```python
from build123d import *

# Parameters (mm, degrees)
BASPROSKE_W             = 10
BASPROSKE_H             = 11
TOOTHCUT_DEPTH          = 19.493242009
TEETHCUTS_COUNT         = 20
TEETHCUTS_ANGLE         = 342
BORSKE_R                = 0.4
BORE_DEPTH              = 50.0000508
CROQUIS1_R              = 2
SALIENTE_EXTRUIR1_DEPTH = 10
CROQUIS2_R              = 2
CORTAR_EXTRUIR1_DEPTH   = 10
CORTAR_EXTRUIR2_DEPTH   = 10


with BuildPart() as part:
    # BasProSke → Base-Revolve (revolve)
    with BuildSketch(Plane(origin=(0, 0, 0), x_dir=(1, 0, 0), z_dir=(0, 1, 0)), mode=Mode.PRIVATE) as base_revolve_sk:
        with Locations((5, 5.5)):
            Rectangle(BASPROSKE_W, BASPROSKE_H)
    revolve(base_revolve_sk.sketch.rotate(Axis((-10, 0, 0), (1, 0, 0)), 180), axis=Axis((-10, 0, 0), (1, 0, 0)))

    # TooCutSke → ToothCut (cut, through all)
    with BuildSketch(Plane(origin=(0, 0, 0), x_dir=(0, 0, -1), z_dir=(1, 0, 0))):
        with BuildLine():
            ThreePointArc((0.499924007, 8.734705318), (0, 8.749), (-0.499924007, 8.734705318))
            ThreePointArc((-0.499924007, 8.734705318), (-0.824302243, 9.905497836), (-1.485192705, 10.924909509))
            ThreePointArc((-1.485192705, 10.924909509), (0, 11.0254), (1.485192705, 10.924909509))
            ThreePointArc((1.485192705, 10.924909509), (0.824302243, 9.905497836), (0.499924007, 8.734705318))
        make_face()
    toothcut = extrude(amount=TOOTHCUT_DEPTH, mode=Mode.SUBTRACT)

    # TeethCuts: ToothCut ×20 about axis
    teethcuts_axis = Axis((-10, 0, 0), (1, 0, 0))
    for i in range(1, TEETHCUTS_COUNT):
        add(toothcut.rotate(teethcuts_axis, i * TEETHCUTS_ANGLE / (TEETHCUTS_COUNT - 1)), mode=Mode.SUBTRACT)

    # BorSke → Bore (cut, symmetric)
    with BuildSketch(Plane(origin=(0, 0, 0), x_dir=(0, 0, -1), z_dir=(1, 0, 0))):
        with Locations(Location((0, 0, 0), (0, 0, 180))):
            Circle(BORSKE_R)
    extrude(amount=BORE_DEPTH, both=True, mode=Mode.SUBTRACT)

    # Croquis1 → Saliente-Extruir1 (add)
    with BuildSketch(Plane(origin=(10, 0, 0), x_dir=(0, 0, -1), z_dir=(1, 0, 0))):
        with BuildLine():
            Line((40, 5), (0, 5))
            ThreePointArc((0, 5), (-5, 0), (0, -5))
            Line((0, -5), (40, -5))
            ThreePointArc((40, -5), (45, 0), (40, 5))
        make_face()
        Circle(CROQUIS1_R, mode=Mode.SUBTRACT)
        with Locations((40, 0)):
            Circle(CROQUIS1_R, mode=Mode.SUBTRACT)
    extrude(amount=-SALIENTE_EXTRUIR1_DEPTH)

    # Croquis2 → Cortar-Extruir1 (cut)
    with BuildSketch(Plane(origin=(10, 0, 0), x_dir=(0, 0, -1), z_dir=(1, 0, 0))):
        Circle(CROQUIS2_R)
    extrude(amount=-CORTAR_EXTRUIR1_DEPTH, mode=Mode.SUBTRACT)

    # Croquis3 → Cortar-Extruir2 (cut)
    with BuildSketch(Plane(origin=(10, 0, 0), x_dir=(0, 0, -1), z_dir=(1, 0, 0))):
        with BuildLine():
            Line((6.772677084, 5.538577987), (8.515195785, 6.963579593))
            ThreePointArc((8.515195785, 6.963579593), (9.209061868, 6.016076754), (9.797958971, 5))
            Line((9.797958971, 5), (7.179484731, 5))
            ThreePointArc((7.179484731, 5), (6.981276487, 5.273213405), (6.772677084, 5.538577987))
        make_face()
        with BuildLine():
            Line((6.772677084, -5.538577987), (8.515195785, -6.963579593))
            ThreePointArc((8.515195785, -6.963579593), (9.209061868, -6.016076754), (9.797958971, -5))
            Line((9.797958971, -5), (7.179484731, -5))
            ThreePointArc((7.179484731, -5), (6.981276487, -5.273213405), (6.772677084, -5.538577987))
        make_face()
    extrude(amount=-CORTAR_EXTRUIR2_DEPTH, mode=Mode.SUBTRACT)


solid = part.part
```
Design review of the part built by this model. Coordinates are the model's own, in mm. A direction names the side the tool comes from. Round coordinates to 2 decimals unless told otherwise and drop trailing zeros. Write each loop counter-clockwise with the first axis right and the second up, starting at its lowest first coordinate (ties: lowest second). Pieces come first, ordered by that corner, then holes. Notation, with made-up numbers: (-17, 46.5) -> (4, 46.5) arc R18 cw to (4, 79.5) -> close; hole circle Ø9 at (35, -2). An arc over 180 degrees is marked (long way). Answer in a Markdown table with one row per item.
Q1. Clearance check with flat-ended pins moving along their axes: pin 1 Ø3 at (x, z) = (4, -18.5) entering from -Y; pin 2 Ø3 at (x, y) = (5, -6.5) entering from +Z; pin 3 Ø1 at (x, z) = (6, -15.5) entering from +Y. State where each tip first meets the part, or that it passes through.
The answers:
| item | result |
|---|---|
| pin 1 | y = -5 |
| pin 2 | z = 9.8 |
| pin 3 | y = 5 |
Q2. To check wall thickness, follow L1, parallel to Y at x = 7, z = -40; L2, parallel to Z at x = 0.5, y = 9.5; L3, parallel to Y at x = 5.25, z = 0. State the ranges of each line that lie inside material, in increasing order. Write a range as [from, to].
The answers:
| item | result |
|---|---|
| L1 | [-5, -2], [2, 5] |
| L2 | [-5.24, -4.19], [-2.29, -0.67], [0.67, 2.29], [4.19, 5.24] |
| L3 | [-8.75, -2], [2, 8.75] |
Q3. For faces 1 (the face through (4.93, -7.53, 6.49)), 2 (the face through (4.93, 9.14, 3.82)), 3 (the face through (0, 0, -17)), 4 (the face through (4.93, -3.82, 9.14)), 5 (the face through (4.93, 5.15, 8.47)), list the 3-axis set-ups (+Z, -Z, +X, -X, +Y, -Y) from which the entire face can be reached by the end or side of a thin tool; tool diameter is ignored.
The answers:
| item | result |
|---|---|
| face 1 | +X, -X, -Y |
| face 2 | +X, -X, +Y |
| face 3 | +Z, -Z, -X, +Y, -Y |
| face 4 | +Z, +X, -X |
| face 5 | +X, -X |
Q4. Take a section at D-D, the plane z = -9.5. State the section outline as (x, y) points.
The answers:
| item | result |
|---|---|
| outline | (0, -5) -> (10, -5) -> (10, 5) -> (0, 5) -> close |
Q5. Take a section at A-A, the plane y = 0. State the section outline as (x, z) points, then the cut area to 3 significant figures.
The answers:
| item | result |
|---|---|
| outline | (0, -45) -> (10, -45) -> (10, -42) -> (0, -42) -> close; (0, -38) -> (10, -38) -> (10, -2) -> (0, -2) -> close; (0, 2) -> (10, 2) -> (10, 8.75) -> (0, 8.75) -> close |
| area | 457 mm² |
Q6. Take a section at C-C, the plane x = 7.25. Count the separate pieces of the cut face and the enclosed holes in it, then the cut area to 3 significant figures.
The answers:
| item | result |
|---|---|
| separate pieces | 1 |
| enclosed holes | 2 |
| area | 622 mm² |
Q7. Take a section at B-B, the plane z = -40.5. State the section outline as (x, y) points.
The answers:
| item | result |
|---|---|
| outline | (0, -4.97) -> (10, -4.97) -> (10, -1.94) -> (0, -1.94) -> close; (0, 1.94) -> (10, 1.94) -> (10, 4.97) -> (0, 4.97) -> close |
Q8. Draft analysis for pull direction Y (two halves, no side actions). For faces 6 (the face through (4.93, 9.17, -3.85)), 7 (the face through (4.93, 6.49, 7.53)), 8 (the face through (4.93, -7.513, -6.461)), state which applies: +Y half, -Y half, draft (parallel to the pull), parting line (faces both ways), or undercut.
The answers:
| item | result |
|---|---|
| face 6 | +Y half |
| face 7 | undercut |
| face 8 | -Y half |
